Autodesk Inventor part; units mm, degrees
ref_plane "YZ Plane" through (0, 0, 0) normal (1, 0, 0) x (0, 1, 0)
ref_plane "XZ Plane" through (0, 0, 0) normal (0, 1, 0) x (-1, 0, 0)
ref_plane "XY Plane" through (0, 0, 0) normal (0, 0, 1) x (1, 0, 0)
sketch "Boceto1" plane through (0, 0, 0) normal (0, 1, 0) x (-1, 0, 0)
  line L0 (-7, 3.5) -> (-8.5, 3.5)
  line L1 (-7, -3.5) -> (-7, 3.5)
  line L2 (-8.5, -3.5) -> (-7, -3.5)
  line L3 (-8.5, -3.5) -> (-8.5, -7.3536)
  line L4 (-8.5, -7.3536) -> (8.5, -7.3536)
  line L5 (8.5, -7.3536) -> (8.5, -3.5)
  line L6 (7, -3.5) -> (8.5, -3.5)
  line L7 (7, 3.5) -> (7, -3.5)
  line L8 (8.5, 3.5) -> (7, 3.5)
  line L9 (8.5, 3.5) -> (8.5, 8.8489)
  line L10 (-8.5, 8.8489) -> (8.5, 8.8489)
  line L11 (-8.5, 8.8489) -> (-8.5, 3.5)
  circle A0 centre (0, 0) radius 5.5
  point P0 (-1.5892, 6.097)
  point P1 (-7, 0)
  dimension "d26" = 16.2026
  dimension "d27" = 17
  dimension "d28" = 5.3489
  dimension "d29" = 7
  dimension "d30" = 11
  dimension "d31" = 8.8489
  dimension "d32" = 8.5
  dimension "d34" = 1.5
  dimension "d35" = 1.5
sketch "Boceto2" plane through (0, 0, 0) normal (0, 1, 0) x (-1, 0, 0)
  line L0 (8.5, 3.5) -> (7, 3.5) construction
  line L1 (7, 3.5) -> (7, -3.5) construction
  line L2 (7, -3.5) -> (8.5, -3.5) construction
  line L3 (-7, 3.5) -> (-8.5, 3.5) construction
  line L4 (-7, -3.5) -> (-7, 3.5) construction
  line L5 (-8.5, -3.5) -> (-7, -3.5) construction
  line L6 (-8.5, -3.5) -> (-8.5, -7.3536) construction
  line L7 (-8.5, 8.8489) -> (-8.5, 3.5) construction
  line L8 (8.5, 3.5) -> (8.5, 8.8489) construction
  line L9 (8.5, -7.3536) -> (8.5, -3.5) construction
  line L10 (7, 3.5) -> (8.5, 3.5) construction
  line L11 (8.5, 3.5) -> (8.5, -3.5) construction
  line L12 (8.5, -3.5) -> (7, -3.5) construction
  line L13 (7, -3.5) -> (7, 3.5) construction
  line L14 (-8.5, 3.5) -> (-7, 3.5) construction
  line L15 (-7, 3.5) -> (-7, -3.5) construction
  line L16 (-7, -3.5) -> (-8.5, -3.5) construction
  line L17 (-8.5, -3.5) -> (-8.5, 3.5) construction
  line L18 (7.2, 3.3) -> (8.3, 3.3)
  line L19 (8.3, 3.3) -> (8.3, -3.3)
  line L20 (8.3, -3.3) -> (7.2, -3.3)
  line L21 (7.2, -3.3) -> (7.2, 3.3)
  line L22 (8.5, 8.8489) -> (-8.5, 8.8489)
  line L23 (-8.5, 8.8489) -> (-8.5, -7.3536)
  line L24 (-8.5, -7.3536) -> (8.5, -7.3536)
  line L25 (8.5, -7.3536) -> (8.5, 8.8489)
  line L26 (0, 0) -> (0, -2.5786) construction
  line L27 (-7.2, 3.3) -> (-8.3, 3.3)
  line L28 (-8.3, 3.3) -> (-8.3, -3.3)
  line L29 (-8.3, -3.3) -> (-7.2, -3.3)
  line L30 (-7.2, -3.3) -> (-7.2, 3.3)
  line L31 (8.3, 8.6489) -> (-8.3, 8.6489)
  line L32 (-8.3, 8.6489) -> (-8.3, -7.1536)
  line L33 (-8.3, -7.1536) -> (8.3, -7.1536)
  line L34 (8.3, -7.1536) -> (8.3, 8.6489)
  dimension "d36" = 0.2
  dimension "d41" = 0.2
extrude "Extrusión1" add sketch "Boceto2" against normal blind 1 contours L21 L20 L34 L33 L32 L29 L30 L27 L31 L18 | L18 L19 L20 L21 | L27 L30 L29 L28
extrude "Extrusión2" add sketch "Boceto2" along normal blind 2 contours L18 L19 L20 L21 | L27 L30 L29 L28
chamfer "Chaflán1" distance 1 angle 45 4 edges at (-7.75, 2, 3.3) (-7.75, 2, -3.3) (7.75, 2, 3.3) (7.75, 2, -3.3)
equation "\"d35\" = d34"
properties part number "tapita"
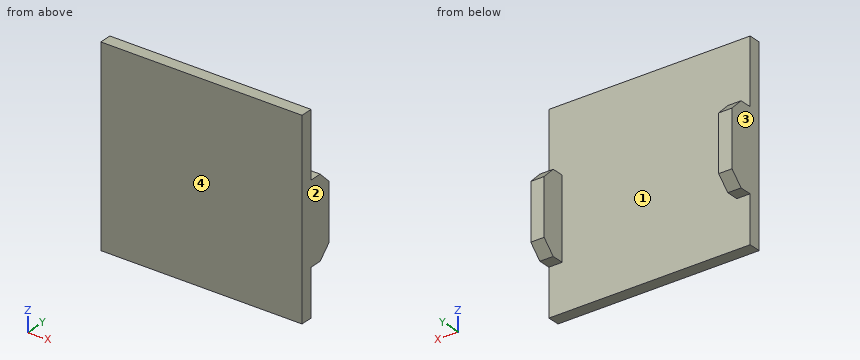
Work out the finished part from the listing and answer in its coordinate system (mm). Face numbers are marked on the shaded views. Round coordinates to 2 decimals unless told otherwise and drop trailing zeros. Loops run counter-clockwise (first coordinate to the right, second up) from the corner with the lowest first, then second, coordinate; pieces in that order, holes last. Notation, with made-up numbers: (72.25, 89.5) - (127.25, 89.5) arc R17 ccw to (127.25, 117.5) - close; hole circle Ø6 at (30, 72.25). An arc over 180 degrees is marked (long way). One line per item, written item: value.
Q1. Find section A-A on y = 0.65. Give the vertices of the cut face in (x, z), and give its area (3 significant figures).
Check values:
outline: (-8.3, -3.3) - (-7.2, -3.3) - (-7.2, 3.3) - (-8.3, 3.3) - close; (7.2, -3.3) - (8.3, -3.3) - (8.3, 3.3) - (7.2, 3.3) - close
area: 14.5 mm2
Q2. Each of these flat-tipped pins is pushed along its axis until it touches: pin 1 Ø5 at (x, z) = (-1, -4) entering from +Y; pin 2 Ø0.5 at (x, y) = (-8, 0.5) entering from +Z; pin 3 Ø0.8 at (x, y) = (7.5, 0.5) entering from -Z. Where does it stop, or does it pass through?
Check values:
pin 1: y = 0
pin 2: z = 3.3
pin 3: z = -3.3
Q3. The mould has two halves that part along X. Classify the marked faces 1, 2, 3 and 4: +X half, -X half, draft (parallel to the pull), parting line (faces both ways), or undercut.
Check values:
face 1: undercut
face 2: +X half
face 3: -X half
face 4: draft
Q4. Find section B-B on z = -2.75. Give the vertices of the cut face in (x, y).
Check values:
outline: (-8.3, -1) - (8.3, -1) - (8.3, 1.55) - (7.2, 1.55) - (7.2, 0) - (-7.2, 0) - (-7.2, 1.55) - (-8.3, 1.55) - close
Q5. Straight lines are drawn through the part: probe 1 along X at (y, z) = (1.4, 0.25); probe 2 along Y at (x, z) = (-3.75, 3.5). For each, find the intervals that lie inside material, in ascending order.
Check values:
probe 1: -8.3 to -7.2, 7.2 to 8.3
probe 2: -1 to 0
Q6. Find section D-D on y = 1.65. Give the vertices of the cut face in (x, z), and give its area (3 significant figures).
Check values:
outline: (-8.3, -2.65) - (-7.2, -2.65) - (-7.2, 2.65) - (-8.3, 2.65) - close; (7.2, -2.65) - (8.3, -2.65) - (8.3, 2.65) - (7.2, 2.65) - close
area: 11.7 mm2
Q7. Find section C-C on x = -4.25. Give the vertices of the cut face in (y, z), and give its area (3 significant figures).
Check values:
outline: (-1, -7.15) - (0, -7.15) - (0, 8.65) - (-1, 8.65) - close
area: 15.8 mm2
